For this review, take the finished solid that the model builds, in its own axes (mm). A direction names the side the tool comes from. Coordinates: 2 decimals unless noted, no trailing zeros. Write each loop counter-clockwise with the first axis right and the second up, starting at its lowest first coordinate (ties: lowest second). Pieces come first, ordered by that corner, then holes.
```python
from build123d import *

# Parameters (mm, degrees)
F1_DEPTH = 2
F0_R     = 2
F3_DEPTH = 4
F4_COUNT = 16


with BuildPart() as f1:
    # F0 (on Front) → F1 (new body)
    with BuildSketch(Plane.XZ):
        Polygon((-0.7803612881, 11.9231411216), (0, 8), (0.7803612881, 11.9231411216), align=None)
    extrude(amount=-F1_DEPTH)



with BuildPart() as f1b:
    # F0 (on Front) → F1, piece 2 (new body)
    with BuildSketch(Plane.XZ):
        Polygon((3.841828747, 11.3141773817), (3.0614674589, 7.3910362601), (5.283748391, 10.7169147093), align=None)
    extrude(amount=-F1_DEPTH)


with BuildPart() as f1c:
    # F0 (on Front) → F1, piece 3 (new body)
    with BuildSketch(Plane.XZ):
        Polygon((7.8791351816, 8.9827326987), (5.6568542495, 5.6568542495), (8.9827326987, 7.8791351816), align=None)
    extrude(amount=-F1_DEPTH)


with BuildPart() as f1d:
    # F0 (on Front) → F1, piece 4 (new body)
    with BuildSketch(Plane.XZ):
        Polygon((10.7169147093, 5.283748391), (7.3910362601, 3.0614674589), (11.3141773817, 3.841828747), align=None)
    extrude(amount=-F1_DEPTH)


with BuildPart() as f1e:
    # F0 (on Front) → F1, piece 5 (new body)
    with BuildSketch(Plane.XZ):
        Polygon((11.9231411216, 0.7803612881), (8, 0), (11.9231411216, -0.7803612881), align=None)
    extrude(amount=-F1_DEPTH)


with BuildPart() as f1f:
    # F0 (on Front) → F1, piece 6 (new body)
    with BuildSketch(Plane.XZ):
        Polygon((11.3141773817, -3.841828747), (7.3910362601, -3.0614674589), (10.7169147093, -5.283748391), align=None)
    extrude(amount=-F1_DEPTH)


with BuildPart() as f1g:
    # F0 (on Front) → F1, piece 7 (new body)
    with BuildSketch(Plane.XZ):
        Polygon((8.9827326987, -7.8791351816), (5.6568542495, -5.6568542495), (7.8791351816, -8.9827326987), align=None)
    extrude(amount=-F1_DEPTH)


with BuildPart() as f1h:
    # F0 (on Front) → F1, piece 8 (new body)
    with BuildSketch(Plane.XZ):
        Polygon((5.283748391, -10.7169147093), (3.0614674589, -7.3910362601), (3.841828747, -11.3141773817), align=None)
    extrude(amount=-F1_DEPTH)


with BuildPart() as f1i:
    # F0 (on Front) → F1, piece 9 (new body)
    with BuildSketch(Plane.XZ):
        Polygon((0.7803612881, -11.9231411216), (0, -8), (-0.7803612881, -11.9231411216), align=None)
    extrude(amount=-F1_DEPTH)


with BuildPart() as f1j:
    # F0 (on Front) → F1, piece 10 (new body)
    with BuildSketch(Plane.XZ):
        Polygon((-3.841828747, -11.3141773817), (-3.0614674589, -7.3910362601), (-5.283748391, -10.7169147093), align=None)
    extrude(amount=-F1_DEPTH)


with BuildPart() as f1k:
    # F0 (on Front) → F1, piece 11 (new body)
    with BuildSketch(Plane.XZ):
        Polygon((-7.8791351816, -8.9827326987), (-5.6568542495, -5.6568542495), (-8.9827326987, -7.8791351816), align=None)
    extrude(amount=-F1_DEPTH)


with BuildPart() as f1l:
    # F0 (on Front) → F1, piece 12 (new body)
    with BuildSketch(Plane.XZ):
        Polygon((-10.7169147093, -5.283748391), (-7.3910362601, -3.0614674589), (-11.3141773817, -3.841828747), align=None)
    extrude(amount=-F1_DEPTH)


with BuildPart() as f1m:
    # F0 (on Front) → F1, piece 13 (new body)
    with BuildSketch(Plane.XZ):
        Polygon((-11.9231411216, -0.7803612881), (-8, 0), (-11.9231411216, 0.7803612881), align=None)
    extrude(amount=-F1_DEPTH)


with BuildPart() as f1n:
    # F0 (on Front) → F1, piece 14 (new body)
    with BuildSketch(Plane.XZ):
        Polygon((-11.3141773817, 3.841828747), (-7.3910362601, 3.0614674589), (-10.7169147093, 5.283748391), align=None)
    extrude(amount=-F1_DEPTH)


with BuildPart() as f1o:
    # F0 (on Front) → F1, piece 15 (new body)
    with BuildSketch(Plane.XZ):
        Polygon((-8.9827326987, 7.8791351816), (-5.6568542495, 5.6568542495), (-7.8791351816, 8.9827326987), align=None)
    extrude(amount=-F1_DEPTH)


with BuildPart() as f1p:
    # F0 (on Front) → F1, piece 16 (new body)
    with BuildSketch(Plane.XZ):
        Polygon((0, 8), (-3.0614674589, 7.3910362601), (-5.6568542495, 5.6568542495), (-7.3910362601, 3.0614674589), (-8, 0), (-7.3910362601, -3.0614674589), (-5.6568542495, -5.6568542495), (-3.0614674589, -7.3910362601), (0, -8), (3.0614674589, -7.3910362601), (5.6568542495, -5.6568542495), (7.3910362601, -3.0614674589), (8, 0), (7.3910362601, 3.0614674589), (5.6568542495, 5.6568542495), (3.0614674589, 7.3910362601), align=None)
        Circle(F0_R, mode=Mode.SUBTRACT)
    extrude(amount=-F1_DEPTH)


with BuildPart() as f1q:
    # F0 (on Front) → F1, piece 17 (new body)
    with BuildSketch(Plane.XZ):
        Polygon((-5.283748391, 10.7169147093), (-3.0614674589, 7.3910362601), (-3.841828747, 11.3141773817), align=None)
    extrude(amount=-F1_DEPTH)


with BuildPart() as f1_1:
    add(f1.part)

    add(f1p.part)  # F3 merges F1p

    add(f1q.part)  # F3 merges F1q
    # F2 (on face) → F3 (join)
    with BuildSketch(Plane(origin=(-1.5307337295, 0, 7.69551813), x_dir=(0.9807852804, 0, 0.195090322), z_dir=(-0.195090322, 0, 0.9807852804))):
        Polygon((-1.5607225761, 2), (-1.5607225761, 0), (0, -2.7032507984), (1.5607225761, 0), (1.5607225761, 2), align=None)
    extrude(amount=F3_DEPTH)



with BuildPart() as f1_2:
    add(f1_1.part)

    add(f1b.part)  # F4 merges F1b

    add(f1c.part)  # F4 merges F1c

    add(f1d.part)  # F4 merges F1d

    add(f1e.part)  # F4 merges F1e

    add(f1f.part)  # F4 merges F1f

    add(f1g.part)  # F4 merges F1g

    add(f1h.part)  # F4 merges F1h

    add(f1i.part)  # F4 merges F1i

    add(f1j.part)  # F4 merges F1j

    add(f1k.part)  # F4 merges F1k

    add(f1l.part)  # F4 merges F1l

    add(f1m.part)  # F4 merges F1m

    add(f1n.part)  # F4 merges F1n

    add(f1o.part)  # F4 merges F1o
    # F4: F1 ×16 about axis
    f4_axis = Axis((0, 0, 0), (0, -1, 0))
    for i in range(1, F4_COUNT):
        add(f1_1.part.rotate(f4_axis, i * 360 / F4_COUNT))


solid = f1_2.part
```
1) Tool access review of faces 4 (the face through (-4.38, -1.03, 6.51)), 5 (the face through (2.29, 0.204, 11.623)), 6 (the face through (-9.78, -1.37, -1.16)): name each direction out of +Z, -Z, +X, -X, +Y, -Y from which nothing blocks a thin tool from reaching the whole face with its end or side.
2) The part is to be moulded in two halves that separate along Z. For faces 1 (the face through (-9.838, 0.204, -6.6)), 2 (the face through (-11, 1, 4.6)), 3 (the face through (7.72, -1.33, 6.11)), say which applies: pulls with the +Z half, pulls with the -Z half, needs draft (parallel to the pull), parting line crosses it, or undercut.
3) For L1, parallel to X at y = 0.65, z = 0; L2, parallel to Z at x = 6.75, y = -0.9, list the stretches that pass through material, from the lowest coordinate up.
4) Clearance check with flat-ended pins moving along their axes: P1, Ø0.8, axis at x = -9, z = 0, coming from the -Y side; P2, Ø0.7, axis at x = 3.5, z = 10, coming from the -Y side; P3, Ø2.5, axis at x = 4.5, z = -8.5, coming from the -Y side. State where each tip first meets the part, or that it passes through.
5) Consider section D-D (y = -1.05). Count the separate pieces of the cut face and the enclosed holes in it, then the cut area to 3 significant figures.
6) Consider section C-C (x = 7). Give the boundary of the cut face in (y, z).
7) Consider section B-B (z = 9.5). Give the boundary of the cut face in (x, y).
Results:
1. face 4: -Y
1. face 5: +Z, +X, +Y, -Y
1. face 6: -X, -Y
2. face 1: pulls with the -Z half
2. face 2: pulls with the +Z half
2. face 3: undercut
3. L1: x = -11.92 to -2, 2 to 11.92
3. L2: z = -9.74 to -8.23, -5.76 to -4.02, 4.02 to 5.76, 8.23 to 9.74
4. P1: stops at y = -0.35
4. P2: stops at y = -0.74
4. P3: stops at y = -2.7
5. separate pieces: 16
5. enclosed holes: 0
5. area: 122 mm2
6. outline: (-2.7, -4.68) - (0, -6.55) - (0, -7.67) - (-1.83, -9.57) - (2, -9.57) - (2, 9.57) - (-1.83, 9.57) - (0, 7.67) - (0, 6.55) - (-2.7, 4.68) - (-1.22, 3.65) - (0, 3.65) - (0, -3.65) - (-1.22, -3.65) - close
7. outline: (-7.1, -1.61) - (-6.35, -2.7) - (-4.47, 0) - (-3.48, 0) - (-1.89, -2.7) - (-0.3, 0) - (0.3, 0) - (1.89, -2.7) - (3.48, 0) - (4.47, 0) - (6.35, -2.7) - (7.1, -1.61) - (7.1, 2) - (-7.1, 2) - close
